Build history of the part. All positions in model axes, mm. A direction names the side the tool comes from. Give positions to 0.01 mm unless a question says otherwise; leave off trailing zeros. Order: outer loops, then holes, each group sorted by start corner. A loop starts at its lowest first (then second) coordinate and runs counter-clockwise, first axis right, second up. Notation, with made-up numbers: M 64.5,50 L 113.5,50 A11 cw 113.5,68 Z; hole C -9,83 d4. An arc over 180 degrees is marked long. One line per item, written item: value. Start each with the question number.
from build123d import *

# Parameters (mm, degrees)
BOSS_EXTRUDE1_DEPTH = 52
BOSS_EXTRUDE3_START = 52
BOSS_EXTRUDE3_DEPTH = 6
CUT_EXTRUDE5_DEPTH  = 76
SKETCH9_W           = 5
SKETCH9_H           = 28
SKETCH9_R           = 7.85
SKETCH9_R_2         = 1.65
CUT_EXTRUDE6_DEPTH  = 21
SKETCH14_R          = 11.5
SKETCH14_R_2        = 1.65
SKETCH14_R_3        = 3
SKETCH14_R_4        = 1.95
CUT_EXTRUDE7_DEPTH  = 62
SKETCH25_R          = 3
CUT_EXTRUDE8_DEPTH  = 3.5
SKETCH26_R          = 6
CUT_EXTRUDE9_DEPTH  = 4
CUT_EXTRUDE10_START = -4
SKETCH27_R          = 6
CUT_EXTRUDE10_DEPTH = 4
SKETCH34_R          = 3
CUT_EXTRUDE11_DEPTH = 4
CUT_EXTRUDE12_START = -4
SKETCH35_R          = 3
CUT_EXTRUDE12_DEPTH = 4
SKETCH36_R          = 4
CUT_EXTRUDE13_DEPTH = 3
SKETCH37_R          = 1.5
CUT_EXTRUDE14_DEPTH = 5
SKETCH38_R          = 1.6
CUT_EXTRUDE15_DEPTH = 4
CUT_EXTRUDE16_START = -6
CUT_EXTRUDE16_DEPTH = 40


with BuildPart() as part:
    # Sketch1 → Boss-Extrude1 (new body)
    with BuildSketch(Plane.XY):
        Polygon((30.491678964, -20.046069124), (30.510764774, -22.022810106), (17.5, -35.03357488), (10.9, -35.03357488), (0, -35.03357488), (-12.996622638, -22.036952242), (-12.996622638, 28.963047758), (-16.496801205, 32.463226325), (-22.496801205, 32.463226325), (-25.996979772, 35.963404892), (-25.996979772, 38.463404892), (38.003020228, 38.463404892), (31.992612588, 32.452997252), (28.992612588, 32.452997252), (28.992612588, 14.752997252), (30.491678964, 13.253930876), align=None)
    extrude(amount=BOSS_EXTRUDE1_DEPTH)

    # Sketch1_4 → Boss-Extrude3 (add)
    with BuildSketch(Plane.XY.offset(BOSS_EXTRUDE3_START)):
        Polygon((30.491678964, -20.046069124), (44.987367978, -34.541758139), (44.987367978, -40.541758139), (41.010691743, -44.500692447), (36.910691743, -44.500692447), (10.9, -35.03357488), (17.5, -35.03357488), (30.510764774, -22.022810106), align=None)
    extrude(amount=-BOSS_EXTRUDE3_DEPTH)

    # Sketch8 → Cut-Extrude5 (cut)
    with BuildSketch(Plane(origin=(40.491678964, 0, 0), x_dir=(0, 0, -1), z_dir=(1, 0, 0))):
        Polygon((-46, 32.452997252), (-46, -49.839210224), (-6, -35.03357488), (-6, 32.452997252), align=None)
    extrude(amount=-CUT_EXTRUDE5_DEPTH, mode=Mode.SUBTRACT)

    # Sketch9 → Cut-Extrude6 (cut)
    with BuildSketch(Plane(origin=(0, 38.463404892, 0), x_dir=(1, 0, 0), z_dir=(0, 1, 0))):
        Polygon((38.003020228, 0), (29.003020228, 0), (37.951108861, -13.263925129), (38.003020228, -13.220806137), align=None)
        Polygon((37.951108861, -38.736074871), (29.003020228, -52), (38.003020228, -52), (38.003020228, -38.759111283), align=None)
        with Locations((-23.496979772, -26)):
            Rectangle(SKETCH9_W, SKETCH9_H)
        with Locations(Location((9.503020228, -26, 0), (0, 0, 270))):
            Circle(SKETCH9_R)
        with Locations(Location((-4.002719293, -12.494260479, 0), (0, 0, 270))):
            Circle(SKETCH9_R_2)
        with Locations(Location((23.008759749, -12.494260479, 0), (0, 0, 270))):
            Circle(SKETCH9_R_2)
        with Locations(Location((23.008759749, -39.505739521, 0), (0, 0, 270))):
            Circle(SKETCH9_R_2)
        with Locations(Location((-4.002719293, -39.505739521, 0), (0, 0, 270))):
            Circle(SKETCH9_R_2)
    extrude(amount=-CUT_EXTRUDE6_DEPTH, mode=Mode.SUBTRACT)

    # Sketch14 → Cut-Extrude7 (cut)
    with BuildSketch(Plane.XY.offset(52)):
        with Locations((8.003377362, 13.463404892)):
            Circle(SKETCH14_R)
        with Locations((-7.496403282, -2.036375752)):
            Circle(SKETCH14_R_2)
        with Locations((-7.496403282, 28.963185535)):
            Circle(SKETCH14_R_2)
        with Locations((23.503158005, 28.963185535)):
            Circle(SKETCH14_R_2)
        with Locations((23.503158005, -2.036375752)):
            Circle(SKETCH14_R_2)
        with Locations((8.003377362, -25.536595108)):
            Circle(SKETCH14_R_3)
        with Locations((38.002754428, -37.535489875)):
            Circle(SKETCH14_R_4)
    extrude(amount=-CUT_EXTRUDE7_DEPTH, mode=Mode.SUBTRACT)

    # Sketch25 → Cut-Extrude8 (cut)
    with BuildSketch(Plane.XZ.offset(-32.452997252)):
        with Locations((-4.002719293, 39.505739521)):
            Circle(SKETCH25_R)
        with Locations((23.008759749, 39.505739521)):
            Circle(SKETCH25_R)
        with Locations((23.008759749, 12.494260479)):
            Circle(SKETCH25_R)
        with Locations((-4.002719293, 12.494260479)):
            Circle(SKETCH25_R)
    extrude(amount=-CUT_EXTRUDE8_DEPTH, mode=Mode.SUBTRACT)

    # Sketch26 → Cut-Extrude9 (cut)
    with BuildSketch(Plane(origin=(0, 0, 0), x_dir=(-1, 0, 0), z_dir=(0, 0, -1))):
        with Locations((-8.003377362, -25.536595108)):
            Circle(SKETCH26_R)
    extrude(amount=-CUT_EXTRUDE9_DEPTH, mode=Mode.SUBTRACT)

    # Sketch27 → Cut-Extrude10 (cut)
    with BuildSketch(Plane.XY.offset(52).offset(CUT_EXTRUDE10_START)):
        with Locations(Location((8.003377362, -25.536595108, 0), (0, 0, 180))):
            Circle(SKETCH27_R)
    extrude(amount=CUT_EXTRUDE10_DEPTH, mode=Mode.SUBTRACT)

    # Sketch34 → Cut-Extrude11 (cut)
    with BuildSketch(Plane(origin=(0, 0, 46), x_dir=(-1, 0, 0), z_dir=(0, 0, -1))):
        with Locations((-23.503158005, 28.963185535)):
            Circle(SKETCH34_R)
        with Locations((7.496403282, 28.963185535)):
            Circle(SKETCH34_R)
        with Locations((7.496403282, -2.036375752)):
            Circle(SKETCH34_R)
        with Locations((-23.503158005, -2.036375752)):
            Circle(SKETCH34_R)
    extrude(amount=-CUT_EXTRUDE11_DEPTH, mode=Mode.SUBTRACT)

    # Sketch35 → Cut-Extrude12 (cut)
    with BuildSketch(Plane.XY.offset(6).offset(CUT_EXTRUDE12_START)):
        with Locations(Location((-7.496403282, 28.963185535, 0), (0, 0, 180))):
            Circle(SKETCH35_R)
        with Locations(Location((23.503158005, -2.036375752, 0), (0, 0, 180))):
            Circle(SKETCH35_R)
        with Locations(Location((-7.496403282, -2.036375752, 0), (0, 0, 180))):
            Circle(SKETCH35_R)
        with Locations(Location((23.503158005, 28.963185535, 0), (0, 0, 180))):
            Circle(SKETCH35_R)
    extrude(amount=CUT_EXTRUDE12_DEPTH, mode=Mode.SUBTRACT)

    # Sketch36 → Cut-Extrude13 (cut)
    with BuildSketch(Plane(origin=(0, 0, 46), x_dir=(-1, 0, 0), z_dir=(0, 0, -1))):
        with Locations((-38.002754428, -37.535489875)):
            Circle(SKETCH36_R)
    extrude(amount=-CUT_EXTRUDE13_DEPTH, mode=Mode.SUBTRACT)

    # Sketch37 → Cut-Extrude14 (cut)
    with BuildSketch(Plane(origin=(30.491678964, 0, 0), x_dir=(0, 0, -1), z_dir=(1, 0, 0))):
        with Locations(Location((-3, 9.953930876, 0), (0, 0, 90))):
            Circle(SKETCH37_R)
        with Locations(Location((-3, -0.046069124, 0), (0, 0, 90))):
            Circle(SKETCH37_R)
        with Locations(Location((-49, 9.953930876, 0), (0, 0, 90))):
            Circle(SKETCH37_R)
        with Locations(Location((-49, -0.046069124, 0), (0, 0, 90))):
            Circle(SKETCH37_R)
    extrude(amount=-CUT_EXTRUDE14_DEPTH, mode=Mode.SUBTRACT)

    # Sketch38 → Cut-Extrude15 (cut)
    with BuildSketch(Plane.ZY.offset(12.996622638)):
        with Locations(Location((49, 13.963047758, 0), (0, 0, 270))):
            Circle(SKETCH38_R)
        with Locations(Location((49, 3.963047758, 0), (0, 0, 270))):
            Circle(SKETCH38_R)
        with Locations(Location((3, 13.963047758, 0), (0, 0, 270))):
            Circle(SKETCH38_R)
        with Locations(Location((3, 3.963047758, 0), (0, 0, 270))):
            Circle(SKETCH38_R)
    extrude(amount=-CUT_EXTRUDE15_DEPTH, mode=Mode.SUBTRACT)

    # Sketch39 → Cut-Extrude16 (cut)
    with BuildSketch(Plane.XY.offset(12).offset(CUT_EXTRUDE16_START)):
        Polygon((-22.496979772, 38.463404892), (-25.996979772, 38.463404892), (-28.276459711, 32.970357014), (-19.102709926, 28.692570726), (-16.496801205, 32.463226325), (-20.996979772, 38.463404892), align=None)
    extrude(amount=CUT_EXTRUDE16_DEPTH, mode=Mode.SUBTRACT)


solid = part.part
1) Slice it at A-A (y = -18). List the corners of the cut face in (x, z).
2) Pull direction Y, two halves, no side cores. Call faces 5 (the flat face through (13, -2, 6)), 6 (the cylindrical face through (22.194, -3.04, 1.014)), 7 (the flat face through (-6.407, -28.626, 2.958)): pulls with the +Y half, pulls with the -Y half, needs draft (parallel to the pull), parting line crosses it, or undercut.
3) Tool access for faces 1 (the cylindrical face through (24.39, 34.18, 9.83)), 2 (the cylindrical face through (-11.025, 3.103, 50.349)), 3 (the flat face through (-9, 30, 2)), 4 (the cylindrical face through (28.03, 10.65, 1.67)): list every direction of +Z, -Z, +X, -X, +Y, -Y with a clear straight run to the whole face (end or side of a thin tool).
4) Drill centre lines: line 1 (Z direction, x = 19, y = 28.5); line 2 (Z direction, x = 22.5, y = -4.5); line 3 (Y direction, x = 0.5, z = 41.5). Where is each one in solid material? Low to high.
5) Drop flat-ended pins along their axis: P1, Ø6.5, axis at y = 3.5, z = 47.5, coming from the +X side; P2, Ø5, axis at y = 13.5, z = 46, coming from the -X side; P3, Ø5.5, axis at x = 23.01, z = 12.49, coming from the +Y side; P4, Ø2.5, axis at y = 3.96, z = 49, coming from the -X side. Give the stop position or say it passes through.
6) Slice it at D-D (x = 33). List the corners of the cut face in (y, z), plus the area to 3 significant figures.
7) Slice it at B-B (y = 19). List the corners of the cut face in (x, z).
Results list:
1. outline: M -13,0 L 30.49,0 L 30.49,6 L -13,6 Z; M -13,46 L 30.49,46 L 30.49,52 L -13,52 Z
2. face 5: needs draft
2. face 6: undercut
2. face 7: pulls with the -Y half
3. face 1: -Y
3. face 2: -X
3. face 3: none
3. face 4: +X
4. line 1: z = 0 to 6, 46 to 52
4. line 2: z = 0 to 2, 50 to 52
4. line 3: y = 32.45 to 38.46
5. P1: stops at x = 30.49
5. P2: stops at x = -13
5. P3: stops at y = 38.46
5. P4: stops at x = -9
6. outline: M -43.08,46 L -22.55,46 L -22.55,52 L -43.08,52 Z; M 33.46,5.92 L 38.46,5.92 L 38.46,46.08 L 33.46,46.08 Z
6. area: 324 mm²
7. outline: M -13,0 L -2.08,0 L -2.08,6 L -13,6 Z; M -13,46 L -2.08,46 L -2.08,52 L -13,52 Z; M 18.08,0 L 28.99,0 L 28.99,6 L 18.08,6 Z; M 18.08,46 L 28.99,46 L 28.99,52 L 18.08,52 Z
